Work out the finished part from the listing and answer in its coordinate system (mm). A direction names the side the tool comes from. Round coordinates to 2 decimals unless told otherwise and drop trailing zeros. Order: outer loops, then holes, each group sorted by start corner. A loop starts at its lowest first (then second) coordinate and runs counter-clockwise, first axis right, second up. Notation, with made-up numbers: (77.25, 12) - (97.25, 12) arc R27 cw to (97.25, 28) - close; hole circle Ø1 at (-12, -25). An arc over 180 degrees is marked (long way). Answer in a Markdown table with one row per item.
from build123d import *

# Parameters (mm, degrees)
F0_R        = 1.625
F1_DEPTH    = 10
F2_W        = 7.875
F2_H        = 2
F2_H_2      = 4
F2_W_2      = 3.5925165284
F1_FACE1_W  = 25
F1_FACE1_H  = 10
F3_DEPTH    = 25
F4_T1_DEPTH = 25
F4_T4_ANGLE = 180
F4_T6_ANGLE = 180


# Not quite as in the source:
# - a fillet or chamfer that OpenCascade refuses, or shapes differently, is made with other operations: its cross-section is extruded or revolved along the edge and cut away or added


with BuildPart() as f1:
    # F0 (on Front) → F1 (new body)
    with BuildSketch(Plane.XZ):
        with BuildLine():
            ThreePointArc((0, -3.5), (2.4748737342, -2.4748737342), (3.5, 0))
            ThreePointArc((3.5, 0), (2.4748737342, 2.4748737342), (0, 3.5))
            ThreePointArc((0, 3.5), (-3.5, 0), (0, -3.5))
        make_face()
        Circle(F0_R, mode=Mode.SUBTRACT)
        with BuildLine():
            ThreePointArc((0, 3.5), (2.4748737342, 2.4748737342), (3.5, 0))
            Line((3.5, 0), (21.5, 0))
            ThreePointArc((21.5, 0), (22.5251262658, 2.4748737342), (25, 3.5))
            Line((25, 3.5), (0, 3.5))
        make_face()
        with BuildLine():
            Line((21.5, 0), (3.5, 0))
            ThreePointArc((3.5, 0), (2.4748737342, -2.4748737342), (0, -3.5))
            Line((0, -3.5), (25, -3.5))
            ThreePointArc((25, -3.5), (22.5251262658, -2.4748737342), (21.5, 0))
        make_face()
        with BuildLine():
            ThreePointArc((25, 3.5), (22.5251262658, 2.4748737342), (21.5, 0))
            ThreePointArc((21.5, 0), (22.5251262658, -2.4748737342), (25, -3.5))
            ThreePointArc((25, -3.5), (27.4748737342, -2.4748737342), (28.5, 0))
            ThreePointArc((28.5, 0), (27.4748737342, 2.4748737342), (25, 3.5))
        make_face()
        with BuildLine():
            ThreePointArc((26.625, 0), (25, -1.625), (23.375, 0))
            ThreePointArc((23.375, 0), (25, 1.625), (26.625, 0))
        make_face(mode=Mode.SUBTRACT)
    extrude(amount=F1_DEPTH)

    # F2 (on face) + F1_face1 (on face) → F3 (cut)
    with BuildSketch(Plane.XY.offset(3.5)):
        with Locations((3.9375, -5)):
            Rectangle(F2_W, F2_H)
        with Locations((3.9375, -2)):
            Rectangle(F2_W, F2_H_2)
        with Locations((11.8125, -5)):
            Rectangle(F2_W, F2_H)
        with Locations((-1.7962582642, -2)):
            Rectangle(F2_W_2, F2_H_2)
        with Locations((-1.7962582642, -5)):
            Rectangle(F2_W_2, F2_H)
        with Locations((11.8125, -2)):
            Rectangle(F2_W, F2_H_2)
        with BuildLine():
            Line((21.75, 0), (15.75, 0))
            Line((15.75, 0), (15.75, -4))
            Line((15.75, -4), (20.75, -4))
            ThreePointArc((20.75, -4), (21.4934164903, -2.5811388301), (21.75, -1))
            Line((21.75, -1), (21.75, 0))
        make_face()
        with BuildLine():
            Line((20.75, -4), (15.75, -4))
            Line((15.75, -4), (15.75, -6))
            Line((15.75, -6), (16.75, -6))
            ThreePointArc((16.75, -6), (18.9860679775, -5.472135955), (20.75, -4))
        make_face()
    with BuildSketch(Plane(origin=(12.5, -5, -3.5), x_dir=(1, 0, 0), z_dir=(0, 0, -1))):
        Rectangle(F1_FACE1_W, F1_FACE1_H)
    extrude(amount=-F3_DEPTH, dir=(0, 0, 1), mode=Mode.SUBTRACT)

    # F4: chamfer of 1 on 6 edges, made by hand

    # F4_s2 → F4_t1 (cut)
    with BuildSketch(Plane.YZ):
        Polygon((-9, 3.5), (-10, 2.5), (-10, 3.5), align=None)
        Polygon((-10, -2.5), (-9, -3.5), (-10, -3.5), align=None)
    extrude(amount=F4_T1_DEPTH, mode=Mode.SUBTRACT)

    # F4_s3 → F4_t4 (revolve, cut)
    with BuildSketch(Plane.YZ):
        Polygon((-9, 3.5), (-10, 2.5), (-10, 3.5), align=None)
    revolve(axis=Axis((0, -10, 0), (0, -1, 0)), revolution_arc=F4_T4_ANGLE, mode=Mode.SUBTRACT)

    # F4_s5 → F4_t6 (revolve, cut)
    with BuildSketch(Plane.YZ.offset(25)):
        Polygon((-10, -2.5), (-9, -3.5), (-10, -3.5), align=None)
    revolve(axis=Axis((25, -10, 0), (0, -1, 0)), revolution_arc=F4_T6_ANGLE, mode=Mode.SUBTRACT)

    # F4_s7 → F4_t8 (revolve, cut)
    with BuildSketch(Plane.XY):
        Polygon((2.625, -10), (1.625, -9), (1.625, -10), align=None)
    revolve(axis=Axis((0, -10, 0), (0, -1, 0)), mode=Mode.SUBTRACT)

    # F4_s9 → F4_t10 (revolve, cut)
    with BuildSketch(Plane.XY):
        Polygon((22.375, -10), (23.375, -9), (23.375, -10), align=None)
    revolve(axis=Axis((25, -10, 0), (0, 1, 0)), mode=Mode.SUBTRACT)


solid = f1.part
1) Find section C-C, the plane y = -5.5. Give the vertices of the cut face in (x, z) (3 decimals).
Filled in:
| item | result |
|---|---|
| outline | (18.929, -3.5) - (25, -3.5) arc R3.5 ccw to (25, 3.5) - (18.929, 3.5) - close; hole circle Ø3.25 at (25, 0) |
2) Find the intervals of material crossed by probe 1 along Z at (x, y) = (0, -8) (3 decimals); probe 2 along X at (y, z) = (-6.25, 0.5); probe 3 along Y at (x, z) = (12.5, -0.25), in increasing order. Write a range as from..to.
Filled in:
| item | result |
|---|---|
| probe 1 | z = -3.5..-1.625, 1.625..3.5 |
| probe 2 | x = -3.46..-1.55, 1.55..23.45, 26.55..28.46 |
| probe 3 | y = -10..-6 |
3) Find section B-B, the plane y = -2.5. Give the vertices of the cut face in (x, z) (3 decimals).
Filled in:
| item | result |
|---|---|
| outline | (21.52, -3.5) - (25, -3.5) arc R3.5 ccw to (25, 3.5) - (21.52, 3.5) - close; hole circle Ø3.25 at (25, 0) |
4) Find section A-A, the plane y = -7.5. Give the vertices of the cut face in (x, z) (3 decimals).
Filled in:
| item | result |
|---|---|
| outline | (0, -3.5) - (25, -3.5) arc R3.5 ccw to (25, 3.5) - (0, 3.5) arc R3.5 ccw to start; hole circle Ø3.25 at (0, 0); hole circle Ø3.25 at (25, 0) |
5) The mould has two halves that part along X. Classify faces 3 (the face through (24, 0, -2)), 4 (the face through (27.7, -9.8, -0.1)), 5 (the face through (23.5, -4.44, -0.62)): released by +X, released by -X, zero draft, split by the parting line, or undercut.
Filled in:
| item | result |
|---|---|
| face 3 | zero draft |
| face 4 | released by +X |
| face 5 | undercut |
6) Which of the six approach directions +Z, -Z, +X, -X, +Y, -Y give full straight-line access (tool end or side, diameter ignored) to faces 1 (the face through (12.3, -9.5, -3)), 2 (the face through (6, -6, 0))?
Filled in:
| item | result |
|---|---|
| face 1 | -Z, +X, -X, -Y |
| face 2 | +Z, -Z, -X, +Y |
7) Each of these flat-tipped pins is pushed along its axis until it touches: pin 1 (0.5 mm diameter, centred on y = -0.5, z = 1.5, fed in from -X); pin 2 (2 mm diameter, centred on y = -5.5, z = 1, fed in from -X); pin 3 (3.5 mm diameter, centred on x = 0, z = 0, fed in from -Y) (3 decimals). Where does it stop, or does it pass through?
Filled in:
| item | result |
|---|---|
| pin 1 | stops at x = 21.75 |
| pin 2 | stops at x = -3.5 |
| pin 3 | stops at y = -9.125 |
